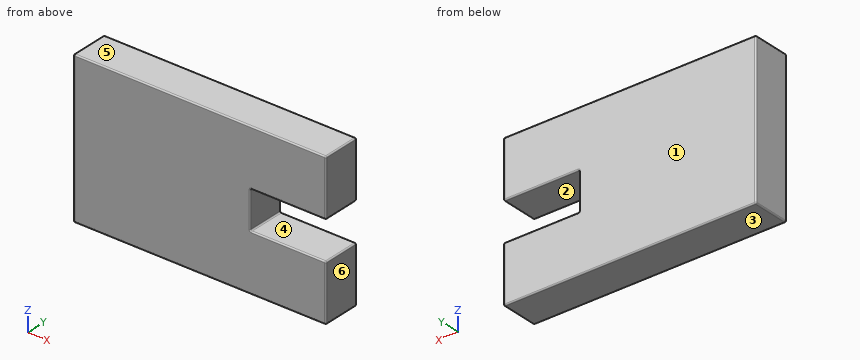
```python
from build123d import *

# Parameters (mm, degrees)
SKETCH1_W           = 200
SKETCH1_H           = 30
BOSS_EXTRUDE1_DEPTH = 60
SKETCH2_W           = 60
SKETCH2_H           = 30
CUT_EXTRUDE2_DEPTH  = 121.415945788
FILLET1_R           = 1


with BuildPart() as part:
    # Sketch1 → Boss-Extrude1 (new, symmetric)
    with BuildSketch(Plane.XY):
        Rectangle(SKETCH1_W, SKETCH1_H)
    extrude(amount=BOSS_EXTRUDE1_DEPTH, both=True)

    # Sketch2 → Cut-Extrude2 (cut, through all)
    with BuildSketch(Plane(origin=(0, 15, 0), x_dir=(1, 0, 0), z_dir=(0, 1, 0))):
        with Locations((70, 0)):
            Rectangle(SKETCH2_W, SKETCH2_H)
    extrude(amount=-CUT_EXTRUDE2_DEPTH, mode=Mode.SUBTRACT)

    # Fillet1
    fillet1_edges = [part.edges().sort_by_distance(p)[0] for p in [
        (-100, 0, 60),
        (100, -15, -37.5),
        (100, 15, -37.5),
        (0, -15, 60),
        (100, 0, -15),
        (70, -15, 15),
        (100, 0, 15),
        (40, -15, 0),
        (40, 0, 15),
        (70, -15, -15),
        (40, 0, -15),
        (70, 15, -15),
        (40, 15, 0),
        (70, 15, 15),
        (100, 0, 60),
        (0, -15, -60),
        (-100, 0, -60),
        (0, 15, -60),
        (100, 0, -60),
        (100, -15, 37.5),
        (-100, -15, 0),
        (-100, 15, 0),
        (100, 15, 37.5),
        (0, 15, 60),
    ]]
    fillet(fillet1_edges, radius=FILLET1_R)


solid = part.part
```
The model under review builds one solid part; all positions refer to its coordinate system, in mm. Face numbers are marked on the shaded views. A direction names the side the tool comes from. Round coordinates to 2 decimals unless told otherwise and drop trailing zeros. Loops run counter-clockwise (first coordinate to the right, second up) from the corner with the lowest first, then second, coordinate; pieces in that order, holes last. Notation, with made-up numbers: M 25,52.5 L 84,52.5 A19 ccw 84,78.5 Z; hole C -24,48.25 d11. An arc over 180 degrees is marked long. Answer as a JSON object with one key per item and string values.
(1) To check wall thickness, follow line 1 along Z through (x, y) = (44, 1); line 2 along X through (y, z) = (-5.5, 12.5). State the ranges of each line that lie inside material, in increasing order.
Resolved:
{"line 1": "-60 to -15, 15 to 60", "line 2": "-100 to 40"}
(2) Clearance check with a flat-ended pin moving along its axis: P1, Ø14, axis at y = 0.5, z = 1, coming from the +X side. State where the tip first meets the part, or that it passes through.
Resolved:
{"P1": "x = 40"}
(3) Draft analysis for pull direction Z (two halves, no side actions). For the marked faces 3, 4, 5 and 6, state which applies: released by +Z, released by -Z, zero draft, split by the parting line, or undercut.
Resolved:
{"face 3": "released by -Z", "face 4": "undercut", "face 5": "released by +Z", "face 6": "zero draft"}
(4) Take a section at A-A on y = -10. Give the boundary of the cut face in (x, z).
Resolved:
{"outline": "M -100,-59 A1 ccw -99,-60 L 99,-60 A1 ccw 100,-59 L 100,-16 A1 ccw 99,-15 L 41,-15 A1 cw 40,-14 L 40,14 A1 cw 41,15 L 99,15 A1 ccw 100,16 L 100,59 A1 ccw 99,60 L -99,60 A1 ccw -100,59 Z"}
(5) Tool access review of the marked faces 1 and 2: name each direction out of +Z, -Z, +X, -X, +Y, -Y from which nothing blocks a thin tool from reaching the whole face with its end or side.
Resolved:
{"face 1": "+Z, -Z, +X, -X, +Y", "face 2": "+X, +Y, -Y"}
(6) Take a section at B-B on z = 8.5. Give the boundary of the cut face in (x, y), and give its area (3 significant figures).
Resolved:
{"outline": "M -100,-14 A1 ccw -99,-15 L 39,-15 A1 ccw 40,-14 L 40,14 A1 ccw 39,15 L -99,15 A1 ccw -100,14 Z", "area": "4,200 mm²"}
